from build123d import *

# Parameters (mm, degrees)
F2_START      = 2
F0_R          = 95
F2_DEPTH      = 23
F4_DEPTH      = 35
F4_DEPTH_BACK = 10
F5_COUNT      = 6
F8_DEPTH      = 8
F8_DEPTH_BACK = 10
F9_COUNT      = 6


with BuildPart() as f2:
    # F0 (on Top) → F2 (new body)
    with BuildSketch(Plane.XY.offset(F2_START)):
        Polygon((75, 129.9038105677), (-75, 129.9038105677), (-150, 0), (-75, -129.9038105677), (75, -129.9038105677), (150, 0), align=None)
        Circle(F0_R, mode=Mode.SUBTRACT)
    extrude(amount=F2_DEPTH)


with BuildPart() as f4:
    # F3 (on Top) → F4 (new body, two sides)
    with BuildSketch(Plane.XY) as f4_sk:
        with BuildLine():
            ThreePointArc((-34.5435296861, 77.6643068393), (-32.6327882373, 78.4863117484), (-30.7025049427, 79.2613158498))
            ThreePointArc((-30.7025049427, 79.2613158498), (-41.9019572207, 106.1559598637), (-65.2675230757, 123.5571075336))
            ThreePointArc((-65.2675230757, 123.5571075336), (-66.656996648, 123.5810891624), (-67.7266746593, 122.6939584625))
            ThreePointArc((-67.7266746593, 122.6939584625), (-67.8817545517, 121.0315856662), (-66.7217246277, 119.8308093913))
            ThreePointArc((-66.7217246277, 119.8308093913), (-44.7195832857, 103.2599332678), (-34.5435296861, 77.6643068393))
        make_face()
    extrude(amount=F4_DEPTH)
    extrude(f4_sk.sketch, amount=-F4_DEPTH_BACK)


with BuildPart() as f5_1:
    # F5: instance of F4
    add(f4.part.rotate(Axis((0, 0, -0.1854561269), (0, 0, 1)), 1 * 360 / F5_COUNT))


with BuildPart() as f5_2:
    # F5: instance of F4
    add(f4.part.rotate(Axis((0, 0, -0.1854561269), (0, 0, 1)), 2 * 360 / F5_COUNT))


with BuildPart() as f5_3:
    # F5: instance of F4
    add(f4.part.rotate(Axis((0, 0, -0.1854561269), (0, 0, 1)), 3 * 360 / F5_COUNT))


with BuildPart() as f5_4:
    # F5: instance of F4
    add(f4.part.rotate(Axis((0, 0, -0.1854561269), (0, 0, 1)), 4 * 360 / F5_COUNT))


with BuildPart() as f5_5:
    # F5: instance of F4
    add(f4.part.rotate(Axis((0, 0, -0.1854561269), (0, 0, 1)), 5 * 360 / F5_COUNT))


with BuildPart() as f2_1:
    add(f2.part)

    # F6: cut F4, F5_5, F5_4, F5_3, F5_2, F5_1
    add(f4.part, mode=Mode.SUBTRACT)
    add(f5_5.part, mode=Mode.SUBTRACT)
    add(f5_4.part, mode=Mode.SUBTRACT)
    add(f5_3.part, mode=Mode.SUBTRACT)
    add(f5_2.part, mode=Mode.SUBTRACT)
    add(f5_1.part, mode=Mode.SUBTRACT)

    # F9: F8 ×6 about axis
    f9_axis = Axis((0, 0, -0.1854561269), (0, 0, 1))


with BuildPart() as f8:
    # F7 (on face) → F8 (new body, two sides)
    with BuildSketch(Plane.XY.offset(25)) as f8_sk:
        with BuildLine():
            ThreePointArc((-14.9635818085, 97.9443271428), (-16.6533189284, 100.4972414515), (-19.6533265238, 101.1075998951))
            ThreePointArc((-19.6533265238, 101.1075998951), (-22.2062408325, 99.4178627752), (-22.8165992761, 96.4178551798))
            Line((-22.8165992761, 96.4178551798), (-20.6971664161, 85.5143183486))
            Line((-20.6971664161, 85.5143183486), (-16.7706576823, 86.2775543301))
            Line((-16.7706576823, 86.2775543301), (-12.8441489485, 87.0407903117))
            Line((-12.8441489485, 87.0407903117), (-14.9635818085, 97.9443271428))
        make_face()
    extrude(amount=-F8_DEPTH)
    extrude(f8_sk.sketch, amount=F8_DEPTH_BACK)


with BuildPart() as f2_2:
    add(f2_1.part)
    for i in range(1, F9_COUNT):
        add(f8.part.rotate(f9_axis, i * 360 / F9_COUNT), mode=Mode.SUBTRACT)

    # F9#seed: cut F8
    add(f8.part, mode=Mode.SUBTRACT)


solid = f2_2.part
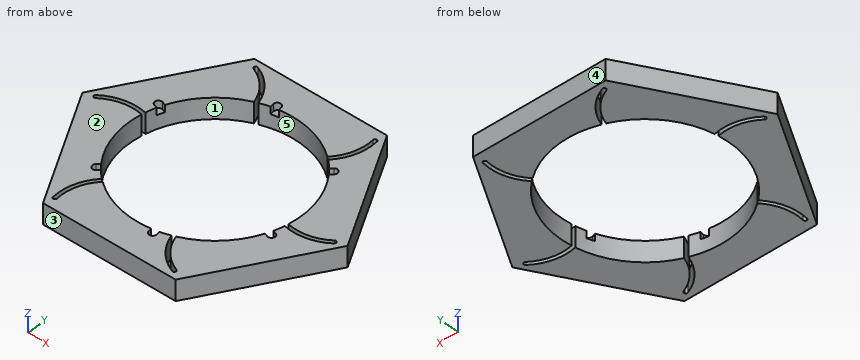
Geometry: final body of the model. Coordinates: model frame, mm. Face numbers are marked on the shaded views. A direction names the side the tool comes from. Coordinates: 2 decimals unless noted, no trailing zeros. Order: outer loops, then holes, each group sorted by start corner. A loop starts at its lowest first (then second) coordinate and runs counter-clockwise, first axis right, second up.
(1) Section query A-A (x = -47.5). Return the cut outline in (y, z).
(2) First-contact query: pin 1 (2.5 mm diameter, centred on x = -17, y = 98.5, fed in from +Z); pin 2 (1 mm diameter, centred on y = -83.5, z = 8.5, fed in from -X); pin 3 (1 mm diameter, centred on y = -58.5, z = 22, fed in from -X). Flat tips, straight axial feed; report the tip coordinate or a pass-through.
(3) Section query D-D (y = 81). Return the cut outline in (x, z).
(4) Section query C-C (x = 85). Return the cut outline in (y, z).
(5) Draft query along Y for the marked faces 1, 2 and 3. Return one class per face: pulls with the +Y half, pulls with the -Y half, needs draft (parallel to the pull), parting line crosses it, or undercut.
(6) Access query for the marked faces 4 and 5. Directions: +Z, -Z, +X, -X, +Y, -Y. A direction counts if a zero-diameter tool reaches every point of the face in a straight line with its end or side. Return the directions, or none.
(7) Section query B-B (y = 51). Return the cut outline in (x, z), plus the area to 3 significant figures.
(8) Material intervals for probe 1 along Y at (x, z) = (-27, 9); probe 2 along Y at (x, z) = (-4.5, 12.75); probe 3 along X at (y, z) = (82, 20.75), sorted ascending.
Solution:
1. outline: (-129.9, 2) - (-82.27, 2) - (-82.27, 25) - (-129.9, 25) - close; (82.27, 2) - (106.6, 2) - (106.6, 25) - (82.27, 25) - close; (112.31, 2) - (129.9, 2) - (129.9, 25) - (112.31, 25) - close
2. pin 1: stops at z = 17
2. pin 2: stops at x = -102.08
2. pin 3: stops at x = -116.51
3. outline: (-103.23, 2) - (-49.64, 2) - (-49.64, 25) - (-103.23, 25) - close; (49.64, 2) - (61.95, 2) - (61.95, 25) - (49.64, 25) - close; (66.73, 2) - (103.23, 2) - (103.23, 25) - (66.73, 25) - close
4. outline: (-112.58, 2) - (-42.43, 2) - (-42.43, 25) - (-112.58, 25) - close; (42.43, 2) - (112.58, 2) - (112.58, 25) - (42.43, 25) - close
5. face 1: undercut
5. face 2: needs draft
5. face 3: pulls with the -Y half
6. face 4: +Z, -Z, +X, -X, +Y
6. face 5: +Z, -Z
7. outline: (-120.56, 2) - (-80.15, 2) - (-80.15, 25) - (-120.56, 25) - close; (80.15, 2) - (120.56, 2) - (120.56, 25) - (80.15, 25) - close
7. area: 1,860 mm2
8. probe 1: y = -129.9 to -91.08, 91.08 to 129.9
8. probe 2: y = -129.9 to -94.89, 94.89 to 129.9
8. probe 3: x = -102.66 to -47.97, 47.97 to 62.63, 67.34 to 102.66
